Input: part model. Units: mm. Frame: model coordinates. Give positions to 0.01 mm unless a question says otherwise; leave off trailing zeros. Loops run counter-clockwise (first coordinate to the right, second up) from the corner with the lowest first, then second, coordinate; pieces in that order, holes last. Notation, with made-up numbers: (73, -7.5) -> (78, -7.5) arc R24 cw to (78, 16.5) -> close; hole circle Ø6 at (54.25, 11). An arc over 180 degrees is marked (long way). One line per question, with ' | ' between items.
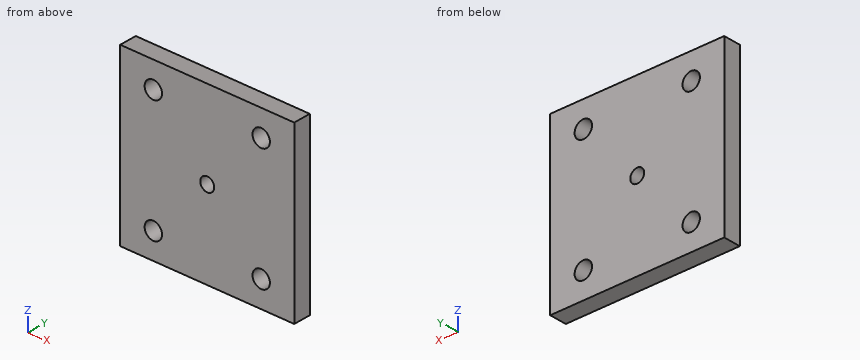
from build123d import *

# Parameters (mm, degrees)
SKETCH1_W           = 50
SKETCH1_H           = 50
BOSS_EXTRUDE1_DEPTH = 5
SKETCH2_R           = 2
CUT_EXTRUDE1_DEPTH  = 5
SKETCH3_R           = 2.5
CUT_EXTRUDE2_DEPTH  = 10


with BuildPart() as part:
    # Sketch1 → Boss-Extrude1 (new body)
    with BuildSketch(Plane(origin=(0, 0, 0), x_dir=(1, 0, 0), z_dir=(0, 1, 0))):
        with Locations((25, 25)):
            Rectangle(SKETCH1_W, SKETCH1_H)
    extrude(amount=BOSS_EXTRUDE1_DEPTH)

    # Sketch2 → Cut-Extrude1 (cut)
    with BuildSketch(Plane(origin=(0, 5, 0), x_dir=(1, 0, 0), z_dir=(0, 1, 0))):
        with Locations(Location((25, 25, 0), (0, 0, 270))):
            Circle(SKETCH2_R)
    extrude(amount=-CUT_EXTRUDE1_DEPTH, mode=Mode.SUBTRACT)

    # Sketch3 → Cut-Extrude2 (cut)
    with BuildSketch(Plane.XZ):
        with Locations(Location((40.5, -42.5, 0), (0, 0, 270))):
            Circle(SKETCH3_R)
        with Locations(Location((9.5, -42.5, 0), (0, 0, 270))):
            Circle(SKETCH3_R)
        with Locations(Location((9.5, -7.5, 0), (0, 0, 270))):
            Circle(SKETCH3_R)
        with Locations(Location((40.5, -7.5, 0), (0, 0, 270))):
            Circle(SKETCH3_R)
    extrude(amount=-CUT_EXTRUDE2_DEPTH, mode=Mode.SUBTRACT)


solid = part.part
1. Section query C-C (x = 9.5). Output: boundary loops of the cut face in (y, z).
Determined:
outline: (0, -50) -> (5, -50) -> (5, -45) -> (0, -45) -> close; (0, -40) -> (5, -40) -> (5, -10) -> (0, -10) -> close; (0, -5) -> (5, -5) -> (5, 0) -> (0, 0) -> close
2. Ray query, line 1 along X through (y, z) = (3.35, -7.5); line 2 along Z through (x, y) = (39, 1.95); line 3 along Z through (x, y) = (40, 4.65). Return the intervals inside material, ascending. Write a range as from..to.
Determined:
line 1: x = 0..7, 12..38, 43..50 | line 2: z = -50..-44.5, -40.5..-9.5, -5.5..0 | line 3: z = -50..-44.95, -40.05..-9.95, -5.05..0
3. Section query D-D (z = -25). Output: boundary loops of the cut face in (x, y).
Determined:
outline: (0, 0) -> (23, 0) -> (23, 5) -> (0, 5) -> close; (27, 0) -> (50, 0) -> (50, 5) -> (27, 5) -> close
4. Section query B-B (y = 0.6). Output: boundary loops of the cut face in (x, z), then the cut area to 3 significant figures.
Determined:
outline: (0, -50) -> (50, -50) -> (50, 0) -> (0, 0) -> close; hole circle Ø5 at (9.5, -42.5); hole circle Ø5 at (9.5, -7.5); hole circle Ø4 at (25, -25); hole circle Ø5 at (40.5, -42.5); hole circle Ø5 at (40.5, -7.5) | area: 2,410 mm2
5. Section query A-A (z = -42.5). Output: boundary loops of the cut face in (x, y).
Determined:
outline: (0, 0) -> (7, 0) -> (7, 5) -> (0, 5) -> close; (12, 0) -> (38, 0) -> (38, 5) -> (12, 5) -> close; (43, 0) -> (50, 0) -> (50, 5) -> (43, 5) -> close
6. Pin query (flat end, axial travel): P1, Ø3, axis at x = 40.5, z = -7.5, coming from the +Y side (1 decimal). Return the tip coordinate at first contact, or that it passes through.
Determined:
P1: passes through
